For this review, take the finished solid that the model builds, in its own axes (mm). A direction names the side the tool comes from. Round coordinates to 2 decimals unless told otherwise and drop trailing zeros. Write each loop counter-clockwise with the first axis right and the second up, starting at its lowest first coordinate (ties: lowest second). Pieces come first, ordered by that corner, then holes. Notation, with made-up numbers: (35, 60.25) -> (87, 60.25) arc R16 ccw to (87, 80.25) -> close; hole circle Ø5 at (-10.5, 24). An arc over 180 degrees is marked (long way). Answer in a Markdown table with one row per item.
from build123d import *

# Parameters (mm, degrees)
BOSS_EXTRUDE1_DEPTH                  = 12.7
M6_CLEARANCE_HOLE1_D                 = 6.4
BOSS_EXTRUDE2_START                  = 11.45
BOSS_EXTRUDE2_DEPTH                  = 11.45
SKETCH2_W                            = 2.5
SKETCH2_H                            = 12.7
TAP_DRILL_FOR_M6X1_0_TAP1_AT_2_COUNT = 2
TAP_DRILL_FOR_M6X1_0_TAP1_AT_2_PITCH = 30
TAP_DRILL_FOR_M6X1_0_TAP1_AT_3_COUNT = 2
TAP_DRILL_FOR_M6X1_0_TAP1_AT_3_PITCH = 51.961524227
TAP_DRILL_FOR_M6X1_0_TAP1_AT_4_COUNT = 2
TAP_DRILL_FOR_M6X1_0_TAP1_AT_4_PITCH = 60
TAP_DRILL_FOR_M6X1_0_TAP1_AT_5_COUNT = 2
TAP_DRILL_FOR_M6X1_0_TAP1_AT_5_PITCH = 51.961524227
TAP_DRILL_FOR_M6X1_0_TAP1_AT_6_COUNT = 2
TAP_DRILL_FOR_M6X1_0_TAP1_AT_6_PITCH = 30
TAP_DRILL_FOR_M6X1_0_TAP3_D          = 5
FILLET1_R                            = 1


with BuildPart() as part:
    # Sketch1 → Boss-Extrude1 (new body)
    with BuildSketch(Plane(origin=(0, 0, 0), x_dir=(1, 0, 0), z_dir=(0, 1, 0))):
        with BuildLine():
            Line((17.139136501, 57.5), (-17.139136501, 57.5))
            ThreePointArc((-17.139136501, 57.5), (-42.426406871, 42.426406871), (-57.5, 17.139136501))
            Line((-57.5, 17.139136501), (-57.5, -17.139136501))
            ThreePointArc((-57.5, -17.139136501), (-42.426406871, -42.426406871), (-17.139136501, -57.5))
            Line((-17.139136501, -57.5), (17.139136501, -57.5))
            ThreePointArc((17.139136501, -57.5), (60, 0), (17.139136501, 57.5))
        make_face()
        with BuildLine():
            Line((-7, 21.38340478), (-7, 29.38340478))
            Line((-7, 29.38340478), (7, 29.38340478))
            Line((7, 29.38340478), (7, 21.38340478))
            ThreePointArc((7, 21.38340478), (0, -22.5), (-7, 21.38340478))
        make_face(mode=Mode.SUBTRACT)
    extrude(amount=-BOSS_EXTRUDE1_DEPTH)

    # M6 Clearance Hole1 (through all)
    with Locations(Plane(origin=(-43.301270189, 0, 25), x_dir=(0, 0, 1), z_dir=(0, 1, 0))):
        with Locations((0, 0), (-75, 43.301270189), (-50, 86.602540378), (0, 86.602540378), (25, 43.301270189), (-50, 0)):
            Hole(M6_CLEARANCE_HOLE1_D / 2)

    # Sketch1<7> → Boss-Extrude2 (add)
    with BuildSketch(Plane(origin=(0, 0, 0), x_dir=(1, 0, 0), z_dir=(0, 1, 0)).offset(BOSS_EXTRUDE2_START)):
        with BuildLine():
            Line((13.919410907, 37.5), (-13.919410907, 37.5))
            ThreePointArc((-13.919410907, 37.5), (-28.284271247, 28.284271247), (-37.5, 13.919410907))
            Line((-37.5, 13.919410907), (-37.5, -13.919410907))
            ThreePointArc((-37.5, -13.919410907), (-28.284271247, -28.284271247), (-13.919410907, -37.5))
            Line((-13.919410907, -37.5), (13.919410907, -37.5))
            ThreePointArc((13.919410907, -37.5), (28.284271247, -28.284271247), (37.5, -13.919410907))
            Line((37.5, -13.919410907), (37.5, 13.919410907))
            ThreePointArc((37.5, 13.919410907), (28.284271247, 28.284271247), (13.919410907, 37.5))
        make_face()
        with BuildLine():
            ThreePointArc((22.5, 0), (-13.205112646, -18.217436702), (-7, 21.38340478))
            Line((-7, 21.38340478), (-7, 29.38340478))
            Line((-7, 29.38340478), (7, 29.38340478))
            Line((7, 29.38340478), (7, 21.38340478))
            ThreePointArc((7, 21.38340478), (18.217436702, 13.205112646), (22.5, 0))
        make_face(mode=Mode.SUBTRACT)
    extrude(amount=-BOSS_EXTRUDE2_DEPTH)

    # Sketch2 → Tap Drill for M6x1.0 Tap1 (revolve, cut)
    with BuildSketch(Plane(origin=(-30, 0, 0), x_dir=(0, 0, 1), z_dir=(1, 0, 0))):
        with Locations((1.25, 6.35)):
            Rectangle(SKETCH2_W, SKETCH2_H)
    tap_drill_for_m6x1_0_tap1 = revolve(axis=Axis((-30, 6.35, 0), (0, -1, 0)), mode=Mode.SUBTRACT)

    # Tap Drill for M6x1.0 Tap1 at 2: Tap Drill for M6x1.0 Tap1 ×2
    with Locations(*[Vector(0.4999999999999998, 0, -0.8660254037844388) * (i * TAP_DRILL_FOR_M6X1_0_TAP1_AT_2_PITCH) for i in range(1, TAP_DRILL_FOR_M6X1_0_TAP1_AT_2_COUNT)]):
        add(tap_drill_for_m6x1_0_tap1, mode=Mode.SUBTRACT)

    # Tap Drill for M6x1.0 Tap1 at 3: Tap Drill for M6x1.0 Tap1 ×2
    with Locations(*[Vector(0.8660254037844386, 0, -0.5000000000000002) * (i * TAP_DRILL_FOR_M6X1_0_TAP1_AT_3_PITCH) for i in range(1, TAP_DRILL_FOR_M6X1_0_TAP1_AT_3_COUNT)]):
        add(tap_drill_for_m6x1_0_tap1, mode=Mode.SUBTRACT)

    # Tap Drill for M6x1.0 Tap1 at 4: Tap Drill for M6x1.0 Tap1 ×2
    with Locations(*[(i * TAP_DRILL_FOR_M6X1_0_TAP1_AT_4_PITCH, 0, 0) for i in range(1, TAP_DRILL_FOR_M6X1_0_TAP1_AT_4_COUNT)]):
        add(tap_drill_for_m6x1_0_tap1, mode=Mode.SUBTRACT)

    # Tap Drill for M6x1.0 Tap1 at 5: Tap Drill for M6x1.0 Tap1 ×2
    with Locations(*[Vector(0.8660254037844388, 0, 0.49999999999999967) * (i * TAP_DRILL_FOR_M6X1_0_TAP1_AT_5_PITCH) for i in range(1, TAP_DRILL_FOR_M6X1_0_TAP1_AT_5_COUNT)]):
        add(tap_drill_for_m6x1_0_tap1, mode=Mode.SUBTRACT)

    # Tap Drill for M6x1.0 Tap1 at 6: Tap Drill for M6x1.0 Tap1 ×2
    with Locations(*[Vector(0.5000000000000006, 0, 0.8660254037844384) * (i * TAP_DRILL_FOR_M6X1_0_TAP1_AT_6_PITCH) for i in range(1, TAP_DRILL_FOR_M6X1_0_TAP1_AT_6_COUNT)]):
        add(tap_drill_for_m6x1_0_tap1, mode=Mode.SUBTRACT)

    # Tap Drill for M6x1.0 Tap3 (through all)
    with Locations(Plane(origin=(30, 0, 0), x_dir=(0, 0, -1), z_dir=(0, -1, 0))):
        with Locations((0, 0), (25.980762114, -45), (-25.980762114, -15), (0, -60), (-25.980762114, -45), (25.980762114, -15)):
            Hole(TAP_DRILL_FOR_M6X1_0_TAP3_D / 2)

    # Fillet1
    fillet1_edges = [part.edges().sort_by_distance(p)[0] for p in [
        (7, -0.625, -21.38340478),
        (7, -0.625, -29.38340478),
        (-7, -0.625, -29.38340478),
        (-7, -0.625, -21.38340478),
    ]]
    fillet(fillet1_edges, radius=FILLET1_R)


solid = part.part
1) Consider section A-A on x = 0. State the section outline as (y, z) points.
Solved:
| item | result |
|---|---|
| outline | (-12.7, -57.5) -> (0, -57.5) -> (0, -53.2) -> (-12.7, -53.2) -> close; (-12.7, -46.8) -> (0, -46.8) -> (0, -37.5) -> (11.45, -37.5) -> (11.45, -29.38) -> (-12.7, -29.38) -> close; (-12.7, 22.5) -> (11.45, 22.5) -> (11.45, 37.5) -> (0, 37.5) -> (0, 46.8) -> (-12.7, 46.8) -> close; (-12.7, 53.2) -> (0, 53.2) -> (0, 57.5) -> (-12.7, 57.5) -> close |
2) For faces 1 (the cylindrical face through (28.113, 5.805, 28.454)), 2 (the flat face through (37.5, 6, 0)), 3 (the flat face through (0, 6, 37.5)), 4 (the cylindrical face through (-28.454, 5.805, 28.113)), 5 (the cylindrical face through (-28.113, 5.805, -28.454)), list the 3-axis set-ups (+Z, -Z, +X, -X, +Y, -Y) from which the entire face can be reached by the end or side of a thin tool; tool diameter is ignored.
Solved:
| item | result |
|---|---|
| face 1 | +Z, +X, +Y |
| face 2 | +Z, -Z, +X, +Y |
| face 3 | +Z, +X, -X, +Y |
| face 4 | +Z, -X, +Y |
| face 5 | -Z, -X, +Y |
3) For line 1 (X direction, y = 4.75, z = 0); line 2 (X direction, y = -8.75, z = -25); line 3 (Z direction, x = -13.5, y = -7), list the stretches that pass through material, from the lowest coordinate up. Write a range as [from, to].
Solved:
| item | result |
|---|---|
| line 1 | [-37.5, -32.5], [-27.5, -22.5], [22.5, 27.5], [32.5, 37.5] |
| line 2 | [-54.54, -46.5], [-40.1, -17.3], [-12.7, -7], [7, 12.7], [17.3, 40.1], [46.5, 54.54] |
| line 3 | [-57.5, -27.98], [-23.98, -18], [18, 23.98], [27.98, 57.5] |
4) Mouldability with a two-part tool opening along X and no side actions: class faces 6 (the flat face through (-7, 0, -25)), 7 (the flat face through (0, -6, 57.5)), 8 (the flat face through (-57.5, -6, 0)) as pulls with the +X half, pulls with the -X half, needs draft (parallel to the pull), parting line crosses it, or undercut.
Solved:
| item | result |
|---|---|
| face 6 | undercut |
| face 7 | needs draft |
| face 8 | pulls with the -X half |
5) Clearance check with flat-ended pins moving along their axes: pin 1 Ø5.5 at (x, y) = (-5.5, 4.5) entering from -Z; pin 2 Ø5 at (x, z) = (-28.5, -37.5) entering from +Y; pin 3 Ø7 at (y, z) = (0, -23.5) entering from -X. State where each tip first meets the part, or that it passes through.
Solved:
| item | result |
|---|---|
| pin 1 | z = -37.5 |
| pin 2 | y = 0 |
| pin 3 | x = -56.57 |
6) Consider section B-B on z = -25. State the section outline as (x, y) points, then the cut area to 3 significant figures.
Solved:
| item | result |
|---|---|
| outline | (-54.54, -12.7) -> (-46.5, -12.7) -> (-46.5, 0) -> (-54.54, 0) -> close; (-40.1, -12.7) -> (-17.3, -12.7) -> (-17.3, 11.45) -> (-31.22, 11.45) -> (-31.22, 0) -> (-40.1, 0) -> close; (-12.7, -12.7) -> (-7, -12.7) -> (-7, 11.45) -> (-12.7, 11.45) -> close; (7, -12.7) -> (12.7, -12.7) -> (12.7, 11.45) -> (7, 11.45) -> close; (17.3, -12.7) -> (40.1, -12.7) -> (40.1, 0) -> (31.22, 0) -> (31.22, 11.45) -> (17.3, 11.45) -> close; (46.5, -12.7) -> (54.54, -12.7) -> (54.54, 0) -> (46.5, 0) -> close |
| area | 1,380 mm² |
7) Consider section C-C on y = 3.5. State the section outline as (x, z) points.
Solved:
| item | result |
|---|---|
| outline | (-37.5, -13.92) arc R40 ccw to (-13.92, -37.5) -> (13.92, -37.5) arc R40 ccw to (37.5, -13.92) -> (37.5, 13.92) arc R40 ccw to (13.92, 37.5) -> (-13.92, 37.5) arc R40 ccw to (-37.5, 13.92) -> close; hole circle Ø5 at (-30, 0); hole circle Ø5 at (-15, -25.98); hole circle Ø5 at (-15, 25.98); hole (-7.66, -21.16) arc R1 cw to (-7, -22.1) -> (-7, -28.38) arc R1 ccw to (-6, -29.38) -> (6, -29.38) arc R1 ccw to (7, -28.38) -> (7, -22.1) arc R1 cw to (7.66, -21.16) arc R22.5 ccw (long way) to start; hole circle Ø5 at (15, -25.98); hole circle Ø5 at (15, 25.98); hole circle Ø5 at (30, 0) |
8) Consider section D-D on x = 30. State the section outline as (y, z) points, then the cut area to 3 significant figures.
Solved:
| item | result |
|---|---|
| outline | (-12.7, -51.96) -> (0, -51.96) -> (0, -26.46) -> (11.45, -26.46) -> (11.45, -2.5) -> (-12.7, -2.5) -> close; (-12.7, 2.5) -> (11.45, 2.5) -> (11.45, 26.46) -> (0, 26.46) -> (0, 51.96) -> (-12.7, 51.96) -> close |
| area | 1,800 mm² |
